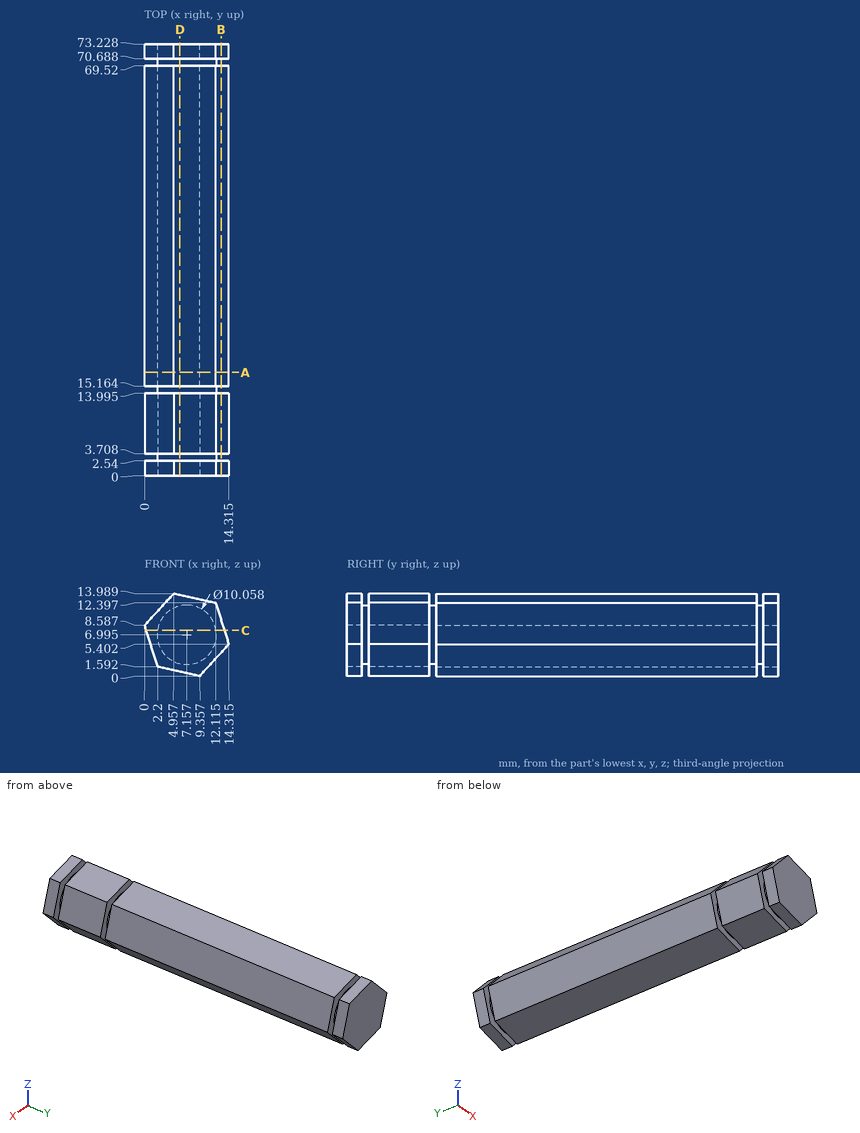
Study the drawing (mm; zero at the part's minimum x, y, z) and answer. Round coordinates to 2 decimals unless told otherwise and drop trailing zeros. Loops run counter-clockwise (first coordinate to the right, second up) from the corner with the lowest first, then second, coordinate; pieces in that order, holes last. Notation, with made-up numbers: (32.5, 62.5) - (65.5, 62.5) arc R23 ccw to (65.5, 81.5) - close; hole circle Ø8 at (18.25, -32.75). An arc over 180 degrees is marked (long way). Use one line per item in the form item = value. Start each with the question number.
1. Consider line 1 (Y direction, x = 13.25, z = 7.5) (1 decimal); line 2 (Z direction, x = 11.5, y = 22) (1 decimal); line 3 (X direction, y = 38.5, z = 2) (1 decimal). Determine where each line is inside the solid, lowest interval first. Write a range as [from, to].
2. Given pin 1 Ø1.5 at (y, z) = (52, 7) entering from +X; pin 2 Ø8 at (y, z) = (8, 11.5) entering from +X (1 decimal); pin 3 Ø1 at (x, y) = (12.5, 63.5) entering from +Z, each flat-ended and moving along its own axis, determine where each tip first touches the part or whether it passes through.
3. The part is cut by section D-D on x = 6. Determine the outline of the cut face in (y, z) (1 decimal).
4. The part is cut by section B-B on x = 13. Determine the outline of the cut face in (y, z) (1 decimal).
5. The part is cut by section C-C on z = 7.75. Determine the outline of the cut face in (x, y) (1 decimal), then the cut area to 3 significant figures.
6. The part is cut by section A-A on y = 17.5. Determine the outline of the cut face in (x, z) (1 decimal), then the cut area to 3 significant figures.
Geometry check:
q1.line_1 = [0, 2.5], [3.7, 14], [15.2, 69.5], [70.7, 73.2]
q1.line_2 = [2.3, 12.5]
q1.line_3 = [2.1, 11.2]
q2.pin_1 = 14.05
q2.pin_2 = 13.7
q2.pin_3 = 12.42
q3.outline = (0, 0.7) - (2.5, 0.7) - (2.5, 2.1) - (3.7, 2.1) - (3.7, 0.7) - (14, 0.7) - (14, 2.1) - (15.2, 2.1) - (15.2, 0.7) - (69.5, 0.7) - (69.5, 2.1) - (70.7, 2.1) - (70.7, 0.7) - (73.2, 0.7) - (73.2, 13.8) - (70.7, 13.8) - (70.7, 11.9) - (69.5, 11.9) - (69.5, 13.8) - (15.2, 13.8) - (15.2, 11.9) - (14, 11.9) - (14, 13.8) - (3.7, 13.8) - (3.7, 11.9) - (2.5, 11.9) - (2.5, 13.8) - (0, 13.8) - close
q4.outline = (0, 4) - (2.5, 4) - (2.5, 9.6) - (0, 9.6) - close; (3.7, 4) - (14, 4) - (14, 9.6) - (3.7, 9.6) - close; (15.2, 4) - (69.5, 4) - (69.5, 9.6) - (15.2, 9.6) - close; (70.7, 4) - (73.2, 4) - (73.2, 9.6) - (70.7, 9.6) - close
q5.outline = (0.3, 0) - (13.6, 0) - (13.6, 2.5) - (12.1, 2.5) - (12.1, 3.7) - (13.6, 3.7) - (13.6, 14) - (12.1, 14) - (12.1, 15.2) - (13.6, 15.2) - (13.6, 69.5) - (12.1, 69.5) - (12.1, 70.7) - (13.6, 70.7) - (13.6, 73.2) - (0.3, 73.2) - (0.3, 70.7) - (2.2, 70.7) - (2.2, 69.5) - (0.3, 69.5) - (0.3, 15.2) - (2.2, 15.2) - (2.2, 14) - (0.3, 14) - (0.3, 3.7) - (2.2, 3.7) - (2.2, 2.5) - (0.3, 2.5) - close
q5.area = 963 mm^2
q6.outline = (0, 8.6) - (2.2, 1.6) - (9.4, 0) - (14.3, 5.4) - (12.1, 12.4) - (5, 14) - close
q6.area = 140 mm^2
